```python
from build123d import *

# Parameters (mm, degrees)
F0_W     = 390.525
F0_H     = 368.3
F1_DEPTH = 19.05
F3_DEPTH = 558.8
F4_W     = 307.975
F4_H     = 533.4
F5_DEPTH = 254


with BuildPart() as f1:
    # F0 (on Front) → F1 (new body)
    with BuildSketch(Plane.XZ):
        Rectangle(F0_W, F0_H)
    extrude(amount=F1_DEPTH)

    # F2 (on face) → F3 (join)
    with BuildSketch(Plane(origin=(0, 0, 0), x_dir=(-1, 0, 0), z_dir=(0, 1, 0))):
        Polygon((-166.6875, -127), (0, -127), (166.6875, -127), (166.6875, 139.7), (-166.6875, 139.7), align=None)
    extrude(amount=F3_DEPTH)

    # F4 (on face) → F5 (cut)
    with BuildSketch(Plane.XY.offset(139.7)):
        with Locations((0, 279.4)):
            Rectangle(F4_W, F4_H)
    extrude(amount=-F5_DEPTH, mode=Mode.SUBTRACT)


solid = f1.part
```
Can you work these out from the model? Positions are in its coordinate system, mm. A direction names the side the tool comes from. Give positions to 0.01 mm unless a question says otherwise; leave off trailing zeros. Loops run counter-clockwise (first coordinate to the right, second up) from the corner with the lowest first, then second, coordinate; pieces in that order, holes last. Notation, with made-up numbers: M -10.5,8.5 L -4.5,8.5 A33 cw -4.5,46.5 Z; hole C 21.25,46 d5. An arc over 180 degrees is marked long. Use CSV: the item, a comma, the result in double quotes. Start each with the question number.
1. On a 3-axis mill with a long thin cutter (end or side, diameter ignored), from which of +Z, -Z, +X, -X, +Y, -Y can I reach the whole of each face in a straight line? I mean faces 4 (the face through (-2, 546.1, 14)), 5 (the face through (-166.688, 275, 4)), 6 (the face through (166.688, 275, 8)), 7 (the face through (-161, 278, 139.7)). Say none if no direction works.
2. Imagine slicing it at B-B, the plane z = 107.5. Write out the boundary of the cut face in (x, y).
3. If I drill on L1, parallel to X at y = 40.5, z = 139.5; L2, parallel to Y at x = -69, z = -41; L3, parallel to Z at x = 86, y = 435, over which ranges is the centre line in solid material (lowest first)?
4. Imagine slicing it at C-C, the plane x = -103.5. Write out the boundary of the cut face in (y, z).
5. Imagine slicing it at A-A, the plane y = 82.5. Write out the boundary of the cut face in (x, z).
6. If we mould it in two halves opening along Y, with no side actions, what happens to faces 1 (the face through (195.262, -9, -3)), 2 (the face through (-2, 283, -114.3)), 3 (the face through (2, 558.8, 8))? For each: released by +Y, released by -Y, zero draft, split by the parting line, or undercut.
7. For P1, Ø3, axis at x = 11.5, y = 290, coming from the -Z side; P2, Ø1, axis at x = 149, y = 247.5, coming from the +Z side; P3, Ø8, axis at y = 59.5, z = -127.5, coming from the +X side, each with a flat end and sliding along its axis, tell me the tip position at first contact or that it passes through.
Response values:
1,face 4,"+Z"
1,face 5,"+Z, -Z, -X, +Y"
1,face 6,"+Z, -Z, +X, +Y"
1,face 7,"+Z, +X, -X, +Y"
2,outline,"M -195.26,-19.05 L 195.26,-19.05 L 195.26,0 L 166.69,0 L 166.69,558.8 L -166.69,558.8 L -166.69,0 L -195.26,0 Z; hole M -153.99,12.7 L 153.99,12.7 L 153.99,546.1 L -153.99,546.1 Z"
3,L1,"-166.69 to -153.99, 153.99 to 166.69"
3,L2,"-19.05 to 12.7, 546.1 to 558.8"
3,L3,"-127 to -114.3"
4,outline,"M -19.05,-184.15 L 0,-184.15 L 0,-127 L 558.8,-127 L 558.8,139.7 L 546.1,139.7 L 546.1,-114.3 L 12.7,-114.3 L 12.7,139.7 L 0,139.7 L 0,184.15 L -19.05,184.15 Z"
5,outline,"M -166.69,-127 L 166.69,-127 L 166.69,139.7 L 153.99,139.7 L 153.99,-114.3 L -153.99,-114.3 L -153.99,139.7 L -166.69,139.7 Z"
6,face 1,"zero draft"
6,face 2,"undercut"
6,face 3,"released by +Y"
7,P1,"z = -127"
7,P2,"z = -114.3"
7,P3,"x = 166.69"
